Can you work these out from the model? Positions are in its coordinate system, mm. Coordinates: 2 decimals unless noted, no trailing zeros. Order: outer loops, then holes, each group sorted by start corner. A loop starts at its lowest first (then second) coordinate and runs counter-clockwise, first axis right, second up. Notation, with made-up numbers: (8.25, 52) -> (43.25, 52) arc R24 ccw to (43.25, 90) -> close; hole circle Ø4 at (-14, 85). An arc over 180 degrees is marked (long way). Answer in a Markdown table with one row per item.
```python
from build123d import *

# Parameters (mm, degrees)
F0_W     = 238.125
F0_H     = 63.5
F1_DEPTH = 50.8
F3_DEPTH = 3.175
F4_W     = 38.1
F4_H     = 19.05
F5_DEPTH = 6.35


with BuildPart() as f1:
    # F0 (on Front) → F1 (new body)
    with BuildSketch(Plane.XZ):
        Rectangle(F0_W, F0_H)
    extrude(amount=F1_DEPTH)

    # F2 (on face) → F3 (join)
    with BuildSketch(Plane.XZ.offset(50.8)):
        Polygon((-87.3125, 0), (-100.0125, 0), (-100.0125, -12.7), (-74.6125, -12.7), (-74.6125, 0), align=None)
        Polygon((-100.0125, 12.7), (-100.0125, 0), (-87.3125, 0), (-74.6125, 0), (-74.6125, 12.7), align=None)
        Polygon((-65.0875, 12.7), (-65.0875, 0), (-52.3875, 0), (-39.6875, 0), (-39.6875, 12.7), align=None)
        Polygon((-52.3875, 0), (-65.0875, 0), (-65.0875, -12.7), (-39.6875, -12.7), (-39.6875, 0), align=None)
        Polygon((-30.1625, 12.7), (-30.1625, 0), (-17.4625, 0), (-4.7625, 0), (-4.7625, 12.7), align=None)
        Polygon((-17.4625, 0), (-30.1625, 0), (-30.1625, -12.7), (-4.7625, -12.7), (-4.7625, 0), align=None)
        Polygon((4.7625, 12.7), (4.7625, 0), (17.4625, 0), (30.1625, 0), (30.1625, 12.7), align=None)
        Polygon((17.4625, 0), (4.7625, 0), (4.7625, -12.7), (30.1625, -12.7), (30.1625, 0), align=None)
        Polygon((39.6875, 12.7), (39.6875, 0), (52.3875, 0), (65.0875, 0), (65.0875, 12.7), align=None)
        Polygon((52.3875, 0), (39.6875, 0), (39.6875, -12.7), (65.0875, -12.7), (65.0875, 0), align=None)
        Polygon((74.6125, 12.7), (74.6125, 0), (87.3125, 0), (100.0125, 0), (100.0125, 12.7), align=None)
        Polygon((87.3125, 0), (74.6125, 0), (74.6125, -12.7), (100.0125, -12.7), (100.0125, 0), align=None)
    extrude(amount=F3_DEPTH)

    # F4 (on face) → F5 (join)
    with BuildSketch(Plane.XY.offset(31.75)):
        with Locations((0, -25.4)):
            Rectangle(F4_W, F4_H)
    extrude(amount=F5_DEPTH)


solid = f1.part
```
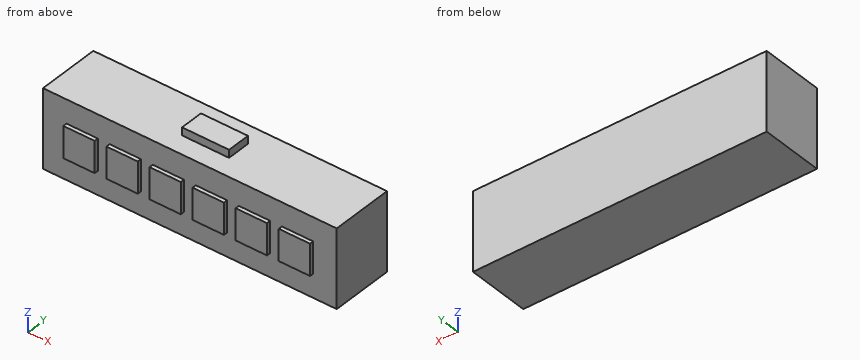
(1) I need wall thicknesses on line 1 (Y direction, x = -84, z = 28); line 2 (Z direction, x = 9.5, y = -51); line 3 (Z direction, x = 58.5, y = -50). Which ranges of each line are inside material? Lowest first, please. Write a range as [from, to].
Response values:
| item | result |
|---|---|
| line 1 | [-50.8, 0] |
| line 2 | [-12.7, 12.7] |
| line 3 | [-31.75, 31.75] |
(2) Suppose I cut it at C-C (y = -23.5). Please give me the cut outline in (x, z).
Response values:
| item | result |
|---|---|
| outline | (-119.06, -31.75) -> (119.06, -31.75) -> (119.06, 31.75) -> (19.05, 31.75) -> (19.05, 38.1) -> (-19.05, 38.1) -> (-19.05, 31.75) -> (-119.06, 31.75) -> close |
(3) Suppose I cut it at A-A (z = 2). Please give me the cut outline in (x, y) (1 decimal), and give its area (3 significant figures).
Response values:
| item | result |
|---|---|
| outline | (-119.1, -50.8) -> (-100, -50.8) -> (-100, -54) -> (-74.6, -54) -> (-74.6, -50.8) -> (-65.1, -50.8) -> (-65.1, -54) -> (-39.7, -54) -> (-39.7, -50.8) -> (-30.2, -50.8) -> (-30.2, -54) -> (-4.8, -54) -> (-4.8, -50.8) -> (4.8, -50.8) -> (4.8, -54) -> (30.2, -54) -> (30.2, -50.8) -> (39.7, -50.8) -> (39.7, -54) -> (65.1, -54) -> (65.1, -50.8) -> (74.6, -50.8) -> (74.6, -54) -> (100, -54) -> (100, -50.8) -> (119.1, -50.8) -> (119.1, 0) -> (-119.1, 0) -> close |
| area | 12,600 mm2 |
(4) Suppose I cut it at D-D (z = 23). Please give me the cut outline in (x, y), and give its area (3 significant figures).
Response values:
| item | result |
|---|---|
| outline | (-119.06, -50.8) -> (119.06, -50.8) -> (119.06, 0) -> (-119.06, 0) -> close |
| area | 12,100 mm2 |
(5) Suppose I cut it at B-B (x = -97). Please give me the cut outline in (y, z) (3 decimals), and give its area (3 significant figures).
Response values:
| item | result |
|---|---|
| outline | (-53.975, -12.7) -> (-50.8, -12.7) -> (-50.8, -31.75) -> (0, -31.75) -> (0, 31.75) -> (-50.8, 31.75) -> (-50.8, 12.7) -> (-53.975, 12.7) -> close |
| area | 3,310 mm2 |
(6) Will these pins go through, and if not, where does the flat tip stop? pin 1 Ø1 at (y, z) = (-52, 5) entering from +X; pin 2 Ø2 at (x, z) = (14, 30) entering from -Y; pin 3 Ø5 at (x, z) = (-9, 34.5) entering from -Y (3 decimals).
Response values:
| item | result |
|---|---|
| pin 1 | x = 100.01 |
| pin 2 | y = -50.8 |
| pin 3 | y = -34.925 |
